Read the model definition and answer for the solid it produces. Units are mm, in the model's axes. Face numbers are marked on the shaded views. A direction names the side the tool comes from. Coordinates: 2 decimals unless noted, no trailing zeros. Order: outer loops, then holes, each group sorted by start corner. A loop starts at its lowest first (then second) coordinate and runs counter-clockwise, first axis right, second up. Notation, with made-up numbers: (-5, 46) -> (47, 46) arc R18 ccw to (47, 71) -> close; hole circle Ø4 at (11, 54.25). An arc over 180 degrees is marked (long way). Answer in a Markdown table with one row per item.
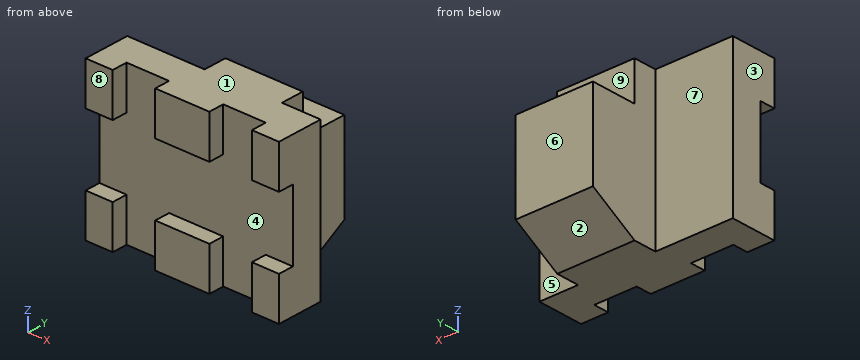
from build123d import *

# Parameters (mm, degrees)
EXTRUDE_1_DEPTH     = 40
SKETCH_2_W          = 18
SKETCH_2_H          = 4
CUT_EXTRUDE_1_DEPTH = 66.76473219
SKETCH_3_W          = 11
SKETCH_3_H          = 4
CUT_EXTRUDE_2_DEPTH = 50.497474683
SKETCH_4_W          = 10
SKETCH_4_H          = 12
CUT_EXTRUDE_3_DEPTH = 59.523499554


with BuildPart() as part:
    # Эскиз1 → Бобышка-Вытянуть1 (new body)
    with BuildSketch(Plane.XY):
        Polygon((-5, -3), (-25, -3), (-25, -15), (25, -15), (25, -3), (15, -3), (15, 15), (-5, 15), align=None)
    extrude(amount=EXTRUDE_1_DEPTH)

    # Эскиз2 → Вырез-Вытянуть1 (cut, through all)
    with BuildSketch(Plane.ZY.offset(25)):
        with Locations((20, -13)):
            Rectangle(SKETCH_2_W, SKETCH_2_H)
    extrude(amount=-CUT_EXTRUDE_1_DEPTH, mode=Mode.SUBTRACT)

    # Эскиз3 → Вырез-Вытянуть2 (cut, through all)
    with BuildSketch(Plane.XY.offset(40)):
        with Locations((-12.5, -13)):
            Rectangle(SKETCH_3_W, SKETCH_3_H)
    cut_extrude_2 = extrude(amount=-CUT_EXTRUDE_2_DEPTH, mode=Mode.SUBTRACT)

    # Зеркальное отражение1: Вырез-Вытянуть2 across plane
    add(cut_extrude_2.mirror(Plane(origin=(0, 0, 0), x_dir=(0, 0, 1), z_dir=(1, 0, 0))), mode=Mode.SUBTRACT)

    # Эскиз4 → Вырез-Вытянуть3 (cut, through all)
    with BuildSketch(Plane(origin=(15, 0, 0), x_dir=(0, 0, -1), z_dir=(1, 0, 0))):
        Polygon((-7, 15), (0, 3), (0, 15), align=None)
        with Locations((-35, 9)):
            Rectangle(SKETCH_4_W, SKETCH_4_H)
    extrude(amount=-CUT_EXTRUDE_3_DEPTH, mode=Mode.SUBTRACT)


solid = part.part
Q1. Given pin 1 (3 mm diameter, centred on y = -0.5, z = 13.5, fed in from -X); pin 2 (5.5 mm diameter, centred on y = 2.5, z = 22.5, fed in from +X); pin 3 (22 mm diameter, centred on x = -17.5, z = 24, fed in from +Y), each flat-ended and moving along its own axis, determine where each tip first touches the part or whether it passes through.
Outcome:
| item | result |
|---|---|
| pin 1 | x = -5 |
| pin 2 | x = 15 |
| pin 3 | y = -3 |
Q2. The part is cut by section A-A (z = 31.5). Write down the section's boundary in (x, y), then the cut area to 3 significant figures.
Outcome:
| item | result |
|---|---|
| outline | (-25, -15) -> (-18, -15) -> (-18, -11) -> (-7, -11) -> (-7, -15) -> (7, -15) -> (7, -11) -> (18, -11) -> (18, -15) -> (25, -15) -> (25, -3) -> (15, -3) -> (15, 3) -> (-5, 3) -> (-5, -3) -> (-25, -3) -> close |
| area | 632 mm² |
Q3. For a pull along Z with two mould halves and no side action, classify the marked faces 1, 2, 3 and 4 as pulls with the +Z half, pulls with the -Z half, needs draft (parallel to the pull), parting line crosses it, or undercut.
Outcome:
| item | result |
|---|---|
| face 1 | pulls with the +Z half |
| face 2 | pulls with the -Z half |
| face 3 | needs draft |
| face 4 | undercut |
Q4. The part is cut by section B-B (x = 3). Write down the section's boundary in (y, z), then the cut area to 3 significant figures.
Outcome:
| item | result |
|---|---|
| outline | (-15, 0) -> (3, 0) -> (15, 7) -> (15, 30) -> (3, 30) -> (3, 40) -> (-15, 40) -> (-15, 29) -> (-11, 29) -> (-11, 11) -> (-15, 11) -> close |
| area | 966 mm² |
Q5. For the marked faces 5, 6, 7, 8 and 9, determine the directions among +Z, -Z, +X, -X, +Y, -Y from which every point of the face is accessible in a straight line to the end or side of a thin tool.
Outcome:
| item | result |
|---|---|
| face 5 | +Z, -Z, +X, +Y |
| face 6 | +Z, -Z, +X, -X, +Y |
| face 7 | +Z, -Z, -X, +Y |
| face 8 | +Z, -Z, +X, -X, -Y |
| face 9 | +Z, +X, -X, +Y |
Q6. The part is cut by section D-D (z = 10). Write down the section's boundary in (x, y).
Outcome:
| item | result |
|---|---|
| outline | (-25, -15) -> (-18, -15) -> (-18, -11) -> (-7, -11) -> (-7, -15) -> (7, -15) -> (7, -11) -> (18, -11) -> (18, -15) -> (25, -15) -> (25, -3) -> (15, -3) -> (15, 15) -> (-5, 15) -> (-5, -3) -> (-25, -3) -> close |
Q7. The part is cut by section C-C (y = -1). Write down the section's boundary in (x, z).
Outcome:
| item | result |
|---|---|
| outline | (-5, 0) -> (15, 0) -> (15, 40) -> (-5, 40) -> close |
Q8. Consider line 1 (X direction, y = -11.5, z = 5); line 2 (Z direction, x = -23, y = -11.75); line 3 (Y direction, x = -10.5, z = 30.5). Determine where each line is inside the solid, lowest interval first.
Outcome:
| item | result |
|---|---|
| line 1 | -25 to -18, -7 to 7, 18 to 25 |
| line 2 | 0 to 11, 29 to 40 |
| line 3 | -11 to -3 |
